Read the model definition and answer for the solid it produces. Units are mm, in the model's axes. Coordinates: 2 decimals unless noted, no trailing zeros. Write each loop counter-clockwise with the first axis right and the second up, starting at its lowest first coordinate (ties: lowest second). Pieces come first, ordered by that corner, then holes. Notation, with made-up numbers: (-28.5, 6) -> (9.5, 6) arc R18 ccw to (9.5, 30) -> close; hole circle Ø9 at (16, -2.5). An arc over 180 degrees is marked (long way). Answer in a Markdown table with one row per item. Add a question column.
Item 1: Given pin 1 Ø3 at (x, y) = (-82.55, 6.35) entering from -Z, flat-ended and moving along its own axis, determine where the tip first touches the part or whether it passes through.
Item 2: Section C-C on y = 6.35 is taken. Write down the section's boundary in (x, z).
Item 3: Straight lines are drawn through the part: line 1 (X direction, y = 6, z = 0.95); line 2 (Y direction, x = 0, z = 1.25); line 3 (X direction, y = 7.5, z = 1.55) (3 decimals). For each, find the intervals that lie inside material, in ascending order. Write a range as from..to.
Item 4: Section A-A on x = 0 is taken. Write down the section's boundary in (y, z), then the cut area to 3 significant figures.
Item 5: Section B-B on z = 2.6 is taken. Write down the section's boundary in (x, y), then the cut area to 3 significant figures.
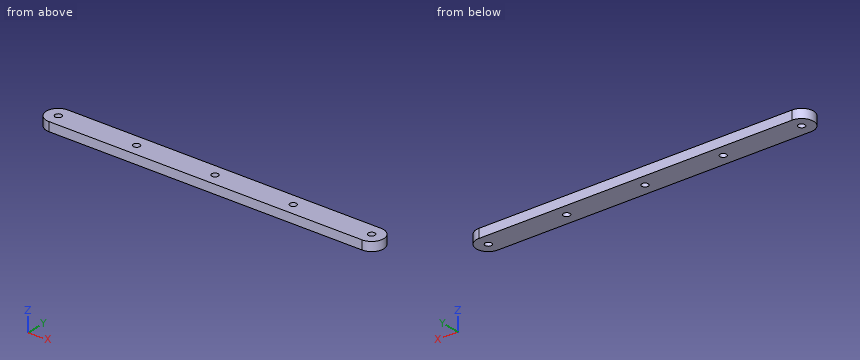
```python
from build123d import *

# Parameters (mm, degrees)
BOSS_EXTRUDE1_DEPTH       = 4.7625
F_8_32_TAPPED_HOLE1_D     = 3.4544
F_8_32_TAPPED_HOLE1_DEPTH = 12.192
F_8_32_TAPPED_HOLE1_TIP   = 1.037806461


with BuildPart() as part:
    # Sketch1 → Boss-Extrude1 (new body)
    with BuildSketch(Plane.XY):
        with BuildLine():
            Line((-82.55, 0), (82.55, 0))
            ThreePointArc((82.55, 0), (88.9, 6.35), (82.55, 12.7))
            Line((82.55, 12.7), (-82.55, 12.7))
            ThreePointArc((-82.55, 12.7), (-88.9, 6.35), (-82.55, 0))
        make_face()
    extrude(amount=BOSS_EXTRUDE1_DEPTH)

    # #8-32 Tapped Hole1
    with Locations(Plane.XY.offset(4.7625)):
        with Locations((-82.55, 6.35), (82.55, 6.35), (0, 6.35), (41.27152138, 6.35), (-41.276070924, 6.35)):
            Hole(F_8_32_TAPPED_HOLE1_D / 2, depth=F_8_32_TAPPED_HOLE1_DEPTH)
            with Locations((0, 0, -(F_8_32_TAPPED_HOLE1_DEPTH + F_8_32_TAPPED_HOLE1_TIP / 2))):  # 118° drill point
                Cone(0, F_8_32_TAPPED_HOLE1_D / 2, F_8_32_TAPPED_HOLE1_TIP, mode=Mode.SUBTRACT)


solid = part.part
```
Results below:
| question | item | result |
|---|---|---|
| 1 | pin 1 | passes through |
| 2 | outline | (-88.9, 0) -> (-84.28, 0) -> (-84.28, 4.76) -> (-88.9, 4.76) -> close; (-80.82, 0) -> (-43, 0) -> (-43, 4.76) -> (-80.82, 4.76) -> close; (-39.55, 0) -> (-1.73, 0) -> (-1.73, 4.76) -> (-39.55, 4.76) -> close; (1.73, 0) -> (39.54, 0) -> (39.54, 4.76) -> (1.73, 4.76) -> close; (43, 0) -> (80.82, 0) -> (80.82, 4.76) -> (43, 4.76) -> close; (84.28, 0) -> (88.9, 0) -> (88.9, 4.76) -> (84.28, 4.76) -> close |
| 3 | line 1 | x = -88.89..-84.24, -80.86..-42.97, -39.58..-1.69, 1.69..39.58, 42.96..80.86, 84.24..88.89 |
| 3 | line 2 | y = 0..4.62, 8.08..12.7 |
| 3 | line 3 | x = -88.795..-83.839, -81.261..-42.565, -39.987..-1.289, 1.289..39.983, 42.56..81.261, 83.839..88.795 |
| 4 | outline | (0, 0) -> (4.62, 0) -> (4.62, 4.76) -> (0, 4.76) -> close; (8.08, 0) -> (12.7, 0) -> (12.7, 4.76) -> (8.08, 4.76) -> close |
| 4 | area | 44.0 mm2 |
| 5 | outline | (-82.55, 0) -> (82.55, 0) arc R6.35 ccw to (82.55, 12.7) -> (-82.55, 12.7) arc R6.35 ccw to start; hole circle Ø3.45 at (-82.55, 6.35); hole circle Ø3.45 at (-41.28, 6.35); hole circle Ø3.45 at (0, 6.35); hole circle Ø3.45 at (41.27, 6.35); hole circle Ø3.45 at (82.55, 6.35) |
| 5 | area | 2,180 mm2 |
